Here's the drawing with two shaded views (mm, measured from the low corner). I have some questions. Give positions to 0.01 mm unless a question says otherwise; leave off trailing zeros. Write each loop counter-clockwise with the first axis right and the second up, starting at its lowest first coordinate (ties: lowest second). Pieces come first, ordered by that corner, then holes.
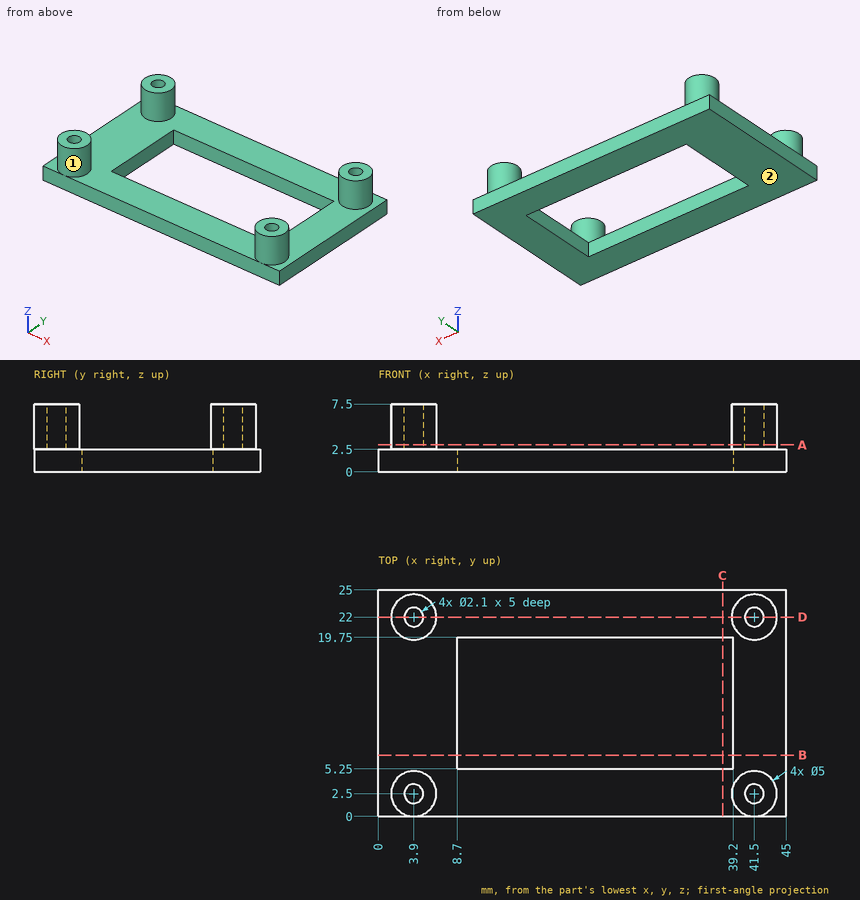
(1) Imagine slicing it at C-C, the plane x = 38. Write out the boundary of the cut face in (y, z), plus the area to 4 significant figures.
Returned:
outline: (0, 0) - (5.25, 0) - (5.25, 2.5) - (0, 2.5) - close; (19.75, 0) - (25, 0) - (25, 2.5) - (19.75, 2.5) - close
area: 26.25 mm2
(2) Will these pins go through, and if not, where does the flat tip stop? P1, Ø0.6, axis at x = 4, y = 22.5, coming from the +Z side; P2, Ø1.5, axis at y = 4, z = 6.5, coming from the -X side; P3, Ø1, axis at x = 13.5, y = 6.5, coming from the -Z side.
Returned:
P1: stops at z = 2.5
P2: stops at x = 1.52
P3: passes through
(3) If we mould it in two halves opening along Y, with no side actions, what happens to the marked faces 1 and 2? For each: +Y half, -Y half, draft (parallel to the pull), parting line (faces both ways), or undercut.
Returned:
face 1: undercut
face 2: draft
(4) Imagine slicing it at D-D, the plane y = 22. Write out the boundary of the cut face in (x, z).
Returned:
outline: (0, 0) - (45, 0) - (45, 2.5) - (44, 2.5) - (44, 7.5) - (42.55, 7.5) - (42.55, 2.5) - (40.45, 2.5) - (40.45, 7.5) - (39, 7.5) - (39, 2.5) - (6.4, 2.5) - (6.4, 7.5) - (4.95, 7.5) - (4.95, 2.5) - (2.85, 2.5) - (2.85, 7.5) - (1.4, 7.5) - (1.4, 2.5) - (0, 2.5) - close
(5) If I drill on L1, parallel to Y at x = 4, z = 5.5; L2, parallel to X at y = 8.5, z = 1; L3, parallel to Y at x = 10.5, z = 2.25, over which ranges is the centre line in solid material (lowest first)?
Returned:
L1: y = 0 to 1.45, 3.55 to 5, 19.5 to 20.95, 23.05 to 24.5
L2: x = 0 to 8.7, 39.2 to 45
L3: y = 0 to 5.25, 19.75 to 25
(6) Imagine slicing it at B-B, the plane y = 6.75. Write out the boundary of the cut face in (x, z), plus the area to 4 significant figures.
Returned:
outline: (0, 0) - (8.7, 0) - (8.7, 2.5) - (0, 2.5) - close; (39.2, 0) - (45, 0) - (45, 2.5) - (39.2, 2.5) - close
area: 36.25 mm2
(7) Imagine slicing it at A-A, the plane z = 3. Write out the boundary of the cut face in (x, y).
Returned:
outline: circle Ø5 at (3.9, 2.5); circle Ø5 at (3.9, 22); circle Ø5 at (41.5, 2.5); circle Ø5 at (41.5, 22); hole circle Ø2.1 at (3.9, 2.5); hole circle Ø2.1 at (3.9, 22); hole circle Ø2.1 at (41.5, 2.5); hole circle Ø2.1 at (41.5, 22)
